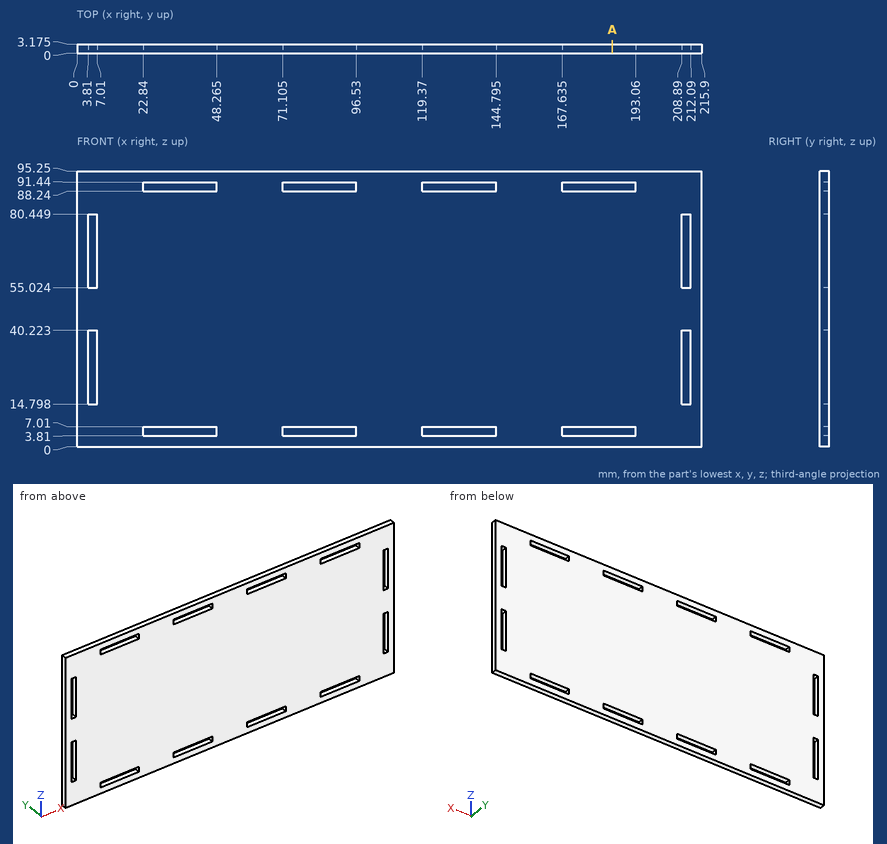
Input: dimensioned drawing with shaded views. Units: mm. Origin: part minimum x, y, z. Give positions to 0.01 mm unless a question says otherwise; leave off trailing zeros. One line per item, written item: value. Start each with the question number.
Q1. Section query A-A, the plane x = 185. Count the separate pieces of the cut face and the enclosed holes in it, then the cut area to 3 significant figures.
Q2. Material intervals for probe 1 along X at (y, z) = (2.4, 72); probe 2 along X at (y, z) = (1.55, 6) (1 decimal); probe 3 along Z at (x, y) = (138, 2.8), sorted ascending. Write a range as from..to.
Q3. First-contact query: pin 1 Ø8 at (x, z) = (182, 56.5) entering from -Y. Flat tip, straight axial feed; report the tip coordinate or a pass-through.
Answer:
1. separate pieces: 3
1. enclosed holes: 0
1. area: 282 mm2
2. probe 1: x = 0..3.81, 7.01..208.89, 212.09..215.9
2. probe 2: x = 0..22.8, 48.3..71.1, 96.5..119.4, 144.8..167.6, 193.1..215.9
2. probe 3: z = 0..3.81, 7.01..88.24, 91.44..95.25
3. pin 1: stops at y = 0
